The model under review builds one solid part; all positions refer to its coordinate system, in mm. Face numbers are marked on the shaded views. A direction names the side the tool comes from. Coordinates: 2 decimals unless noted, no trailing zeros. Order: outer loops, then holes, each group sorted by start corner. A loop starts at its lowest first (then second) coordinate and runs counter-clockwise, first axis right, second up. Notation, with made-up numbers: (41, 72) -> (78, 72) arc R10 cw to (78, 88) -> close; hole circle Ø6 at (20.5, 73). An arc over 180 degrees is marked (long way). Use one line per item in the form item = value.
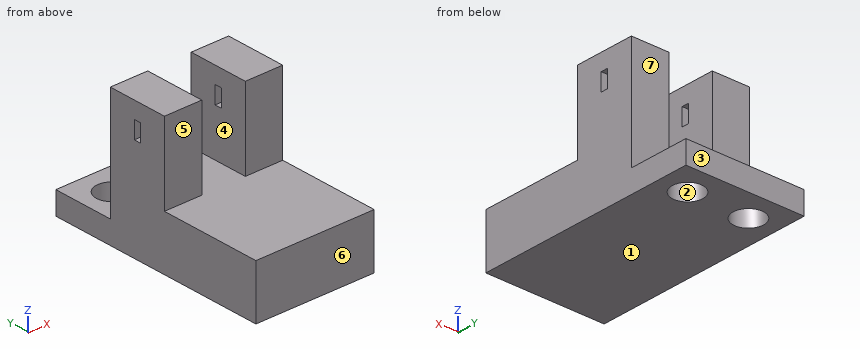
from build123d import *

# Parameters (mm, degrees)
SKETCH_1_W          = 13.6
SKETCH_1_H          = 18.7
EXTRUDE_1_DEPTH     = 6.2
SKETCH_2_W          = 4.3
SKETCH_2_H          = 6.95
EXTRUDE_2_DEPTH     = 9.3
SKETCH_3_W          = 13.6
SKETCH_3_H          = 7
SKETCH_3_R          = 1.75
EXTRUDE_3_DEPTH     = 2.6
SKETCH_4_W          = 2
SKETCH_4_H          = 0.8
CUT_EXTRUDE_1_DEPTH = 26.856720596


with BuildPart() as part:
    # 草图1 → 凸台-拉伸1 (new body)
    with BuildSketch(Plane.XY):
        with Locations((0, -0.75)):
            Rectangle(SKETCH_1_W, SKETCH_1_H)
    extrude(amount=EXTRUDE_1_DEPTH)

    # 草图2 → 凸台-拉伸2 (add)
    with BuildSketch(Plane.XY.offset(6.2)):
        with Locations((4.65, 5.125)):
            Rectangle(SKETCH_2_W, SKETCH_2_H)
        with Locations((-4.65, 5.125)):
            Rectangle(SKETCH_2_W, SKETCH_2_H)
    extrude(amount=EXTRUDE_2_DEPTH)

    # 草图3 → 凸台-拉伸3 (add)
    with BuildSketch(Plane(origin=(0, 0, 0), x_dir=(-1, 0, 0), z_dir=(0, 0, -1))):
        with Locations((0, 12.1)):
            Rectangle(SKETCH_3_W, SKETCH_3_H)
        with Locations((-3.5, 12.125)):
            Circle(SKETCH_3_R, mode=Mode.SUBTRACT)
        with Locations((3.5, 12.125)):
            Circle(SKETCH_3_R, mode=Mode.SUBTRACT)
    extrude(amount=-EXTRUDE_3_DEPTH)

    # 草图4 → 切除-拉伸1 (cut, through all)
    with BuildSketch(Plane(origin=(6.8, 0, 0), x_dir=(0, 0, -1), z_dir=(1, 0, 0))):
        with Locations((-12.6, 5.125)):
            Rectangle(SKETCH_4_W, SKETCH_4_H)
    extrude(amount=-CUT_EXTRUDE_1_DEPTH, mode=Mode.SUBTRACT)


solid = part.part
Item 1: Draft analysis for pull direction Y (two halves, no side actions). For the marked faces 1, 2 and 3, state which applies: released by +Y, released by -Y, zero draft, split by the parting line, or undercut.
Results found:
face_1 = zero draft
face_2 = undercut
face_3 = released by +Y
Item 2: We need section C-C (x = 5.75). Write out the cut boundary in (y, z) (3 decimals).
Results found:
outline = (-10.1, 0) -> (15.6, 0) -> (15.6, 2.6) -> (8.6, 2.6) -> (8.6, 15.5) -> (1.65, 15.5) -> (1.65, 6.2) -> (-10.1, 6.2) -> close; hole (4.725, 11.6) -> (5.525, 11.6) -> (5.525, 13.6) -> (4.725, 13.6) -> close
Item 3: We need section B-B (z = 13). Write out the cut boundary in (x, y) (3 decimals).
Results found:
outline = (-6.8, 1.65) -> (-2.5, 1.65) -> (-2.5, 4.725) -> (-6.8, 4.725) -> close; (-6.8, 5.525) -> (-2.5, 5.525) -> (-2.5, 8.6) -> (-6.8, 8.6) -> close; (2.5, 1.65) -> (6.8, 1.65) -> (6.8, 4.725) -> (2.5, 4.725) -> close; (2.5, 5.525) -> (6.8, 5.525) -> (6.8, 8.6) -> (2.5, 8.6) -> close
Item 4: Tool access review of the marked faces 4, 5, 6 and 7: name each direction out of +Z, -Z, +X, -X, +Y, -Y from which nothing blocks a thin tool from reaching the whole face with its end or side.
Results found:
face_4 = +Z, +Y, -Y
face_5 = +Z, +X, -X, -Y
face_6 = +Z, -Z, +X, -X, -Y
face_7 = +Z, +X, -X, +Y
Item 5: We need section D-D (z = 10.75). Write out the cut boundary in (x, y), plus the area to 3 significant figures.
Results found:
outline = (-6.8, 1.65) -> (-2.5, 1.65) -> (-2.5, 8.6) -> (-6.8, 8.6) -> close; (2.5, 1.65) -> (6.8, 1.65) -> (6.8, 8.6) -> (2.5, 8.6) -> close
area = 59.8 mm²
Item 6: Clearance check with flat-ended pins moving along their axes: pin 1 (2 mm diameter, centred on x = 2.5, z = 8.5, fed in from +Y); pin 2 (7 mm diameter, centred on x = 0.5, y = -2.5, fed in from +Z); pin 3 (5 mm diameter, centred on x = 3.5, z = 13.5, fed in from -Y). State where each tip first meets the part, or that it passes through.
Results found:
pin_1 = 8.6
pin_2 = 6.2
pin_3 = 1.65
Item 7: We need section A-A (x = 3.5). Write out the cut boundary in (y, z) (3 decimals), plus the area to 3 significant figures.
Results found:
outline = (-10.1, 0) -> (10.375, 0) -> (10.375, 2.6) -> (8.6, 2.6) -> (8.6, 15.5) -> (1.65, 15.5) -> (1.65, 6.2) -> (-10.1, 6.2) -> close; (13.875, 0) -> (15.6, 0) -> (15.6, 2.6) -> (13.875, 2.6) -> close; hole (4.725, 11.6) -> (5.525, 11.6) -> (5.525, 13.6) -> (4.725, 13.6) -> close
area = 188 mm²
Item 8: To check wall thickness, follow L1, parallel to Y at x = 3.5, z = 1 (3 decimals); L2, parallel to Z at x = -4.5, y = 5.25; L3, parallel to Y at x = -5.25, z = 13.25 (3 decimals). State the ranges of each line that lie inside material, in increasing order. Write a range as from..to.
Results found:
L1 = -10.1..10.375, 13.875..15.6
L2 = 0..11.6, 13.6..15.5
L3 = 1.65..4.725, 5.525..8.6
